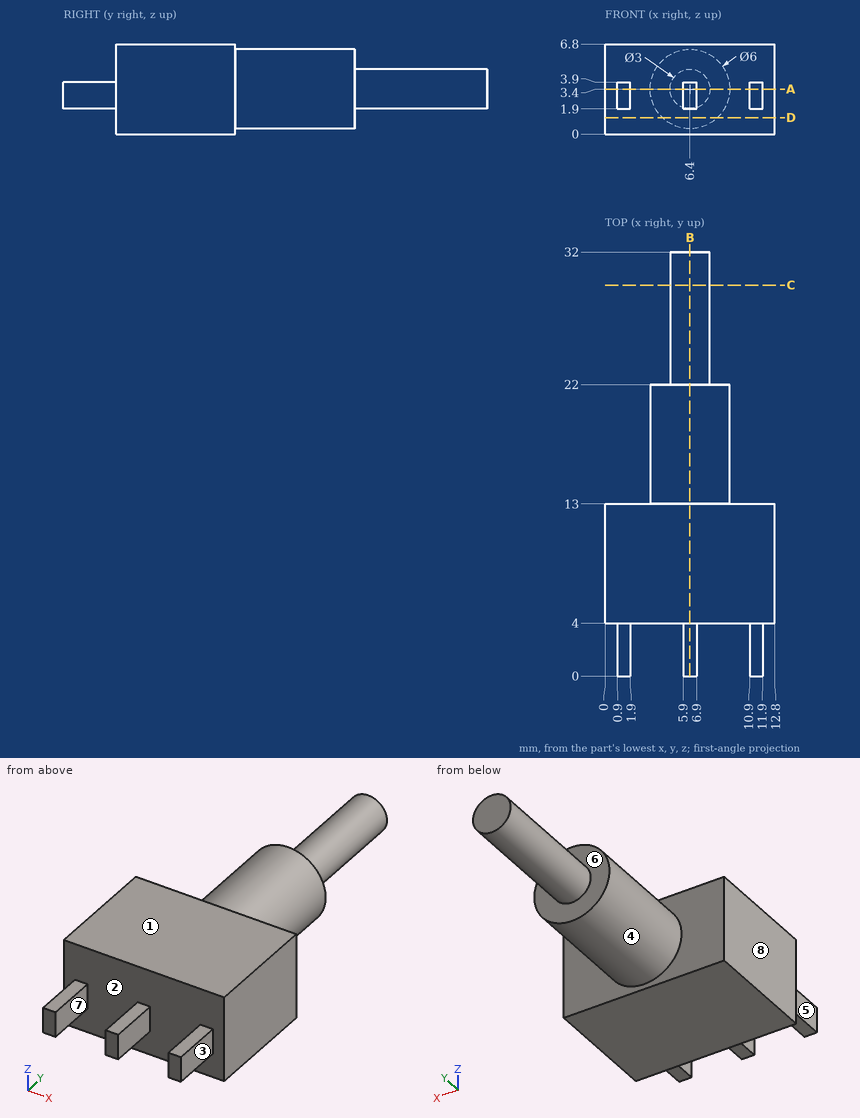
For this review, use the dimensioned drawing (mm, ordinates from the lowest corner) and the shaded views. A direction names the side the tool comes from. Round coordinates to 2 decimals unless told otherwise and drop trailing zeros. Order: outer loops, then holes, each group sorted by start corner. A loop starts at its lowest first (then second) coordinate and runs counter-clockwise, first axis right, second up. Notation, with made-up numbers: (-25, -21.5) -> (18, -21.5) arc R36 cw to (18, 17.5) -> close; hole circle Ø3 at (33, 19). An arc over 180 degrees is marked (long way). Put each result on its own line as item: value.
Q1. Machinability: for the marked faces 5, 6, 7 and 8, which of the approach directions +Z, -Z, +X, -X, +Y, -Y give a long, thin tool a straight path to every point of the face, cutting with its end or side? Answer none if there is none.
Check result:
face 5: +Z, -Z, -X, -Y
face 6: +Y
face 7: +Z, -Z, -Y
face 8: +Z, -Z, -X, +Y, -Y
Q2. For probe 1 along Y at (x, z) = (3.25, 4.25); probe 2 along X at (y, z) = (19.5, 3.5); probe 3 along Y at (x, z) = (5.75, 0.75), list the stretches that pass through material, from the lowest coordinate up. Write a range as [from, to].
Check result:
probe 1: [4, 13]
probe 2: [3.4, 9.4]
probe 3: [4, 22]
Q3. Add section B-B on x = 6.4. Write out the cut boundary in (y, z).
Check result:
outline: (0, 1.9) -> (4, 1.9) -> (4, 0) -> (13, 0) -> (13, 0.4) -> (22, 0.4) -> (22, 1.9) -> (32, 1.9) -> (32, 4.9) -> (22, 4.9) -> (22, 6.4) -> (13, 6.4) -> (13, 6.8) -> (4, 6.8) -> (4, 3.9) -> (0, 3.9) -> close
Q4. Add section C-C on y = 29.5. Write out the cut boundary in (x, z).
Check result:
outline: circle Ø3 at (6.4, 3.4)
Q5. Add section A-A on z = 3.4. Write out the cut boundary in (x, y).
Check result:
outline: (0, 4) -> (0.9, 4) -> (0.9, 0) -> (1.9, 0) -> (1.9, 4) -> (5.9, 4) -> (5.9, 0) -> (6.9, 0) -> (6.9, 4) -> (10.9, 4) -> (10.9, 0) -> (11.9, 0) -> (11.9, 4) -> (12.8, 4) -> (12.8, 13) -> (9.4, 13) -> (9.4, 22) -> (7.9, 22) -> (7.9, 32) -> (4.9, 32) -> (4.9, 22) -> (3.4, 22) -> (3.4, 13) -> (0, 13) -> close
Q6. Add section D-D on z = 1.25. Write out the cut boundary in (x, y).
Check result:
outline: (0, 4) -> (12.8, 4) -> (12.8, 13) -> (8.49, 13) -> (8.49, 22) -> (4.31, 22) -> (4.31, 13) -> (0, 13) -> close
Q7. Mouldability with a two-part tool opening along X and no side actions: class the marked faces 1, 2, 3 and 4 as pulls with the +X half, pulls with the -X half, needs draft (parallel to the pull), parting line crosses it, or undercut.
Check result:
face 1: needs draft
face 2: undercut
face 3: pulls with the +X half
face 4: parting line crosses it
Q8. Insertion check: pin 1 Ø0.8 at (x, y) = (6, 2) entering from +Z; pin 2 Ø6 at (x, y) = (9, 19) entering from -Z; pin 3 Ø4 at (x, y) = (7.5, 28.5) entering from -Z. Each pin has a flat end and moves straight along its axis. Give the tip position at first contact, or say it passes through.
Check result:
pin 1: z = 3.9
pin 2: z = 0.4
pin 3: z = 1.9
